The listing builds one solid part. Answer for the finished solid, in the listing's coordinates (mm). A direction names the side the tool comes from. Coordinates: 2 decimals unless noted, no trailing zeros. Order: outer loops, then holes, each group sorted by start corner. A loop starts at its lowest first (then second) coordinate and runs counter-clockwise, first axis right, second up. Notation, with made-up numbers: (61.5, 57) -> (112.5, 57) arc R9 cw to (112.5, 63) -> close; hole circle Ø6 at (35, -14). An arc over 180 degrees is marked (long way). One line per question, with ' | ' between items.
Autodesk Inventor part; units mm, degrees
ref_plane "YZ Plane" through (0, 0, 0) normal (1, 0, 0) x (0, 1, 0)
ref_plane "XZ Plane" through (0, 0, 0) normal (0, 1, 0) x (-1, 0, 0)
ref_plane "XY Plane" through (0, 0, 0) normal (0, 0, 1) x (1, 0, 0)
sketch "Sketch1" plane through (0, 0, 0) normal (0, 0, 1) x (1, 0, 0)
  circle A0 centre (0, 0) radius 11
  line L0 (-7.7, 0) -> (7.7, 0) construction
  circle A1 centre (-7.7, 0) radius 1.25
  circle A2 centre (7.7, 0) radius 1.25
  dimension "d0" = 22
  dimension "d1" = 15.4
  dimension "d2" = 2.5
  dimension "d3" = 2.5
extrude "Extrusion1" add sketch "Sketch1" along normal blind 5
sketch "Sketch2" plane through (0, 0, 5) normal (0, 0, 1) x (1, 0, 0)
  circle A0 centre (0, 0) radius 11
  arc A1 (6.6742, -8.8894) -> (0, -4) centre (0, -11) ccw
  arc A2 (0, -4) -> (-6.6362, -8.7727) centre (0, -11) ccw
  point P0 (6.6362, -8.7727)
extrude "Extrusion2" cut sketch "Sketch2" against normal blind 10 contours A2 A1 A0 picked at (-1.3613, -8.6538)
equation "\"d0\" = cs_diam"
equation "\"d1\" = cs_holeSpacing"
equation "\"d2\" = cs_holeDiam"
equation "\"d3\" = cs_holeDiam"
equation "\"d4\" = cs_depth"
equation "\"cs_diam\" = 22"
equation "\"cs_holeSpacing\" = 15.4"
equation "\"cs_holeDiam\" = 2.5"
equation "\"cs_depth\" = 5"
properties part number "Caster Spacer 5mm" material "PMMA Plastic"
Item 1: Find the intervals of material crossed by L1, parallel to Y at x = 7.7, z = 1.5; L2, parallel to X at y = -1, z = 2.9; L3, parallel to Y at x = -7.5, z = 3.2, in increasing order.
Computed values:
L1: y = -7.86 to -1.25, 1.25 to 7.86 | L2: x = -10.95 to -8.45, -6.95 to 6.95, 8.45 to 10.95 | L3: y = -8.05 to -1.23, 1.23 to 8.05
Item 2: Section A-A, the plane z = 0.65 is taken. Give the vertices of the cut face in (x, y).
Computed values:
outline: (-6.64, -8.77) arc R7 cw to (0, -4) arc R7 cw to (6.64, -8.77) arc R11 ccw (long way) to start; hole circle Ø2.5 at (-7.7, 0); hole circle Ø2.5 at (7.7, 0)
Item 3: Determine the mould class of faces 1 (the face through (8.89, -0.38, 2.46)), 2 (the face through (4.137, -5.353, 2.535)), 3 (the face through (0, 1, 5)), 4 (the face through (0, 11, 2)) for opening direction Y: pulls with the +Y half, pulls with the -Y half, needs draft (parallel to the pull), parting line crosses it, or undercut.
Computed values:
face 1: undercut | face 2: pulls with the -Y half | face 3: needs draft | face 4: parting line crosses it
Item 4: Section C-C, the plane y = 0 is taken. Give the vertices of the cut face in (x, z), plus the area to 3 significant figures.
Computed values:
outline: (-11, 0) -> (-8.95, 0) -> (-8.95, 5) -> (-11, 5) -> close; (-6.45, 0) -> (6.45, 0) -> (6.45, 5) -> (-6.45, 5) -> close; (8.95, 0) -> (11, 0) -> (11, 5) -> (8.95, 5) -> close | area: 85.0 mm^2
Item 5: Each of these flat-tipped pins is pushed along its axis until it touches: pin 1 Ø1.5 at (y, z) = (-1.5, 3.5) entering from -X; pin 2 Ø2 at (y, z) = (8.5, 2) entering from +X; pin 3 Ø2 at (y, z) = (2, 2.5) entering from +X. Where does it stop, or does it pass through?
Computed values:
pin 1: stops at x = -10.97 | pin 2: stops at x = 8.05 | pin 3: stops at x = 10.95
Item 6: For faces 5 (the face through (0, 1, 0)), 6 (the face through (-4.037, -5.282, 2.535)), determine the directions among +Z, -Z, +X, -X, +Y, -Y from which every point of the face is accessible in a straight line to the end or side of a thin tool.
Computed values:
face 5: -Z, +X, -X, +Y, -Y | face 6: +Z, -Z, -Y
Item 7: Section B-B, the plane x = -7.7 is taken. Give the vertices of the cut face in (y, z).
Computed values:
outline: (-7.86, 0) -> (-1.25, 0) -> (-1.25, 5) -> (-7.86, 5) -> close; (1.25, 0) -> (7.86, 0) -> (7.86, 5) -> (1.25, 5) -> close
Item 8: Section D-D, the plane x = 7.75 is taken. Give the vertices of the cut face in (y, z), plus the area to 3 significant figures.
Computed values:
outline: (-7.81, 0) -> (-1.25, 0) -> (-1.25, 5) -> (-7.81, 5) -> close; (1.25, 0) -> (7.81, 0) -> (7.81, 5) -> (1.25, 5) -> close | area: 65.6 mm^2
